from build123d import *

# Parameters (mm, degrees)
BOSS_EXTRUDE1_DEPTH = 10
CHAMFER1_SIZE       = 0.2
CHAMFER1_SIZE_2     = 0.206341937
CHAMFER2_SIZE       = 0.5


with BuildPart() as part:
    # Sketch1 → Boss-Extrude1 (new body)
    with BuildSketch(Plane(origin=(0, 0, 0), x_dir=(1, 0, 0), z_dir=(0, 1, 0))):
        with BuildLine():
            ThreePointArc((5, 0), (1.227434059, 4.846999652), (-4.397362252, 2.379748983))
            Line((-4.397362252, 2.379748983), (-2.883140649, 1.5))
            ThreePointArc((-2.883140649, 1.5), (0.772105204, 3.156953207), (3.25, 0))
            ThreePointArc((3.25, 0), (0.772105204, -3.156953207), (-2.883140649, -1.5))
            Line((-2.883140649, -1.5), (-4.397362252, -2.379748983))
            ThreePointArc((-4.397362252, -2.379748983), (1.227434059, -4.846999652), (5, 0))
        make_face()
    extrude(amount=BOSS_EXTRUDE1_DEPTH)

    # Chamfer1
    # the kernel refuses this chamfer: 0.206341937, 0.2, 0.191297121 mm, written as the material it takes off along each edge
    with BuildSketch(Plane(origin=(-2.883140649, -0.514336598, -1.5), x_dir=(0.4881882615859918, 0, -0.8727383463843256), z_dir=(0, 1, 0))) as chamfer1_piece_1:
        with BuildLine():
            Line((0.196815803, 0), (CHAMFER1_SIZE * 0.0163116056584, CHAMFER1_SIZE * 0.99986695691))
            Line((CHAMFER1_SIZE * 0.0163116056584, CHAMFER1_SIZE * 0.99986695691), (0, 0))
            ThreePointArc((0, 0), (0.101193556, 0.001489012), (0.196815803, 0))
        make_face()
    extrude(amount=11.028673195, mode=Mode.SUBTRACT)
    with BuildSketch(Plane(origin=(-4.397362252, -0.531068819, -2.379748983), x_dir=(0.4931124519861111, 0, -0.8699655796042999), z_dir=(0, 1, 0))) as chamfer1_piece_2:
        with BuildLine():
            Line((0.196188757, 0), (-CHAMFER1_SIZE_2 * 0.010660935079, -CHAMFER1_SIZE_2 * 0.999943172174))
            Line((-CHAMFER1_SIZE_2 * 0.010660935079, -CHAMFER1_SIZE_2 * 0.999943172174), (0, 0))
            ThreePointArc((0, 0), (0.100953531, 0.000961526), (0.196188757, 0))
        make_face()
    extrude(amount=11.062137639, mode=Mode.SUBTRACT)
    with BuildSketch(Plane(origin=(-4.397362252, -0.520052168, 2.379748983), x_dir=(0.49362201920020077, 0, 0.8696765503109283), z_dir=(0, 1, 0))) as chamfer1_piece_3:
        with BuildLine():
            Line((0.202045895, 0), (-CHAMFER1_SIZE * 0.0100751366451, CHAMFER1_SIZE * 0.999949244523))
            Line((-CHAMFER1_SIZE * 0.0100751366451, CHAMFER1_SIZE * 0.999949244523), (0, 0))
            ThreePointArc((0, 0), (0.103969214, -0.0010198), (0.202045895, 0))
        make_face()
    extrude(amount=11.040104337, mode=Mode.SUBTRACT)
    # the kernel refuses this chamfer: 0.206341937, 0.2, 0.191297121 mm, written as the material it takes off along each edge
    with BuildSketch(Plane(origin=(-2.438414829, 10, 1.241618342), x_dir=(0.502359075260422, 0, 0.8646591001680913), z_dir=(-0.8646591001680916, 0, 0.5023590752604221))) as chamfer1_2_piece_1:
        Polygon((CHAMFER1_SIZE, 0), (0, -CHAMFER1_SIZE), (0, 0), align=None)
    extrude(amount=2.57990857, mode=Mode.SUBTRACT)

    # Chamfer2
    # the kernel refuses this chamfer: 0.5 mm, written as the material it takes off along each edge
    with BuildSketch(Plane(origin=(0, 10, 0), x_dir=(-0.9618869269385497, 0, -0.2734475082803154), z_dir=(-0.2734475082803154, 0, 0.9618869269385497))) as chamfer2_piece_1:
        Polygon((5, CHAMFER2_SIZE), (5 - CHAMFER2_SIZE, 0), (5, 0), align=None)
    revolve(axis=Axis((0, 10, 0), (0, -1, 0)), revolution_arc=328.193834559, mode=Mode.SUBTRACT)


solid = part.part
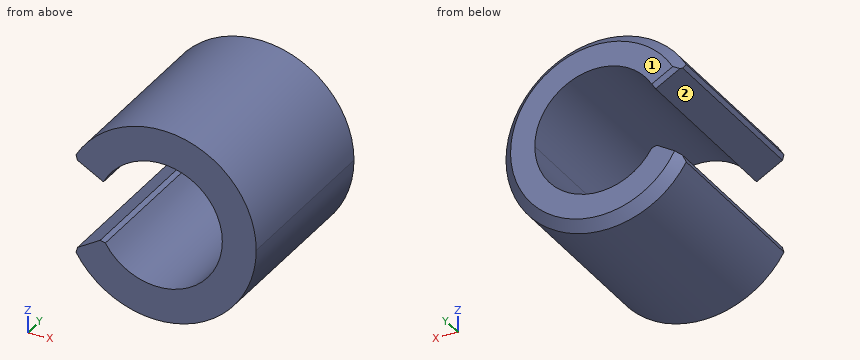
Geometry: final body of the model. Coordinates: model frame, mm. Face numbers are marked on the shaded views. Coordinates: 2 decimals unless noted, no trailing zeros. Loops run counter-clockwise (first coordinate to the right, second up) from the corner with the lowest first, then second, coordinate; pieces in that order, holes last. Notation, with made-up numbers: M 24,82 L 66,82 A16 ccw 66,109 Z; hole C 72.25,-7.75 d1. An arc over 180 degrees is marked long. One line per item, written item: value. Start each with the question number.
1) Material intervals for L1, parallel to Z at x = -1.75, y = 2.5; L2, parallel to Z at x = -3.25, y = 5.5; L3, parallel to X at y = 8, z = -1.75, sorted ascending. Write a range as from..to.
2) Cut plane B-B (y = 9.25). Return loops of the section in (x, z), then the cut area to 3 significant figures.
3) Pin query (flat end, axial travel): P1, Ø2, axis at y = 6.5, z = 1.5, coming from the -X side. Return the tip coordinate at first contact, or that it passes through.
4) Draft query along Z for the marked faces 1 and 2. Return one class per face: released by +Z, released by -Z, zero draft, split by the parting line, or undercut.
5) Cut plane A-A (x = 0). Return loops of the section in (y, z), then the cut area to 4 significant figures.
Evaluation:
1. L1: -4.68..-2.74, 2.74..4.68
1. L2: -3.8..-1.71, 1.71..3.8
1. L3: -3.31..-2.74, 2.74..4.68
2. outline: M -4.3,-2.55 A5 ccw long -4.3,2.56 L -4.22,2.28 L -2.88,1.5 A3.25 cw long -2.79,-1.67 L -3.06,-1.6 L -4.22,-2.28 Z
2. area: 38.2 mm^2
3. P1: x = -4.28
4. face 1: zero draft
4. face 2: undercut
5. outline: M 0,-5 L 9.5,-5 L 10,-4.5 L 10,-3.25 L 0,-3.25 Z; M 0,3.25 L 10,3.25 L 10,4.5 L 9.5,5 L 0,5 Z
5. area: 34.75 mm^2
